```python
from build123d import *

# Parameters (mm, degrees)
F0_R     = 2.25
F0_R_2   = 1.5
F0_R_3   = 3
F0_W     = 71.6
F0_H     = 55.3
F0_W_2   = 30
F0_H_2   = 130
F0_W_3   = 243.84
F0_H_3   = 173
F0_R_4   = 1.75
F1_DEPTH = 3
F2_R     = 10


with BuildPart() as f1:
    # F0 (on Front) → F1 (new body)
    with BuildSketch(Plane.XZ):
        with BuildLine():
            Line((-179.2, 113.305101), (-179.2, 63.305101))
            Line((-179.2, 63.305101), (-163.2, 63.305101))
            Line((-163.2, 63.305101), (-149.2, 63.305101))
            Line((-149.2, 63.305101), (-149.2, 116.305101))
            ThreePointArc((-149.2, 116.305101), (-147.735534, 119.840635), (-144.2, 121.305101))
            Line((-144.2, 121.305101), (-49.2, 121.305101))
            ThreePointArc((-49.2, 121.305101), (-45.664466, 119.840635), (-44.2, 116.305101))
            Line((-44.2, 116.305101), (-44.2, 63.305101))
            Line((-44.2, 63.305101), (-43.607167, 63.305101))
            Line((-43.607167, 63.305101), (-36.2, 63.305101))
            Line((-36.2, 63.305101), (-14.2, 63.305101))
            Line((-14.2, 63.305101), (-14.2, 113.305101))
            ThreePointArc((-14.2, 113.305101), (-18.593398, 123.911702), (-29.2, 128.305101))
            Line((-29.2, 128.305101), (-163.2, 128.305101))
            Line((-163.2, 128.305101), (-164.2, 128.305101))
            ThreePointArc((-164.2, 128.305101), (-174.806602, 123.911702), (-179.2, 113.305101))
        make_face()
        with Locations((-153.7, 70.805101)):
            Circle(F0_R, mode=Mode.SUBTRACT)
        with Locations((-153.704742, 121.805101)):
            Circle(F0_R, mode=Mode.SUBTRACT)
        with Locations((-40.7, 70.805101)):
            Circle(F0_R, mode=Mode.SUBTRACT)
        with Locations((-40.704742, 121.805101)):
            Circle(F0_R, mode=Mode.SUBTRACT)
        with BuildLine():
            Line((-179.2, 63.305101), (-224.2, 63.305101))
            Line((-224.2, 63.305101), (-224.2, -116.694899))
            Line((-224.2, -116.694899), (211.64, -116.694899))
            Line((211.64, -116.694899), (211.64, 63.305101))
            Line((211.64, 63.305101), (-14.2, 63.305101))
            Line((-14.2, 63.305101), (-36.2, 63.305101))
            Line((-36.2, 63.305101), (-36.2, -38.694899))
            Line((-36.2, -38.694899), (-96.871792, -38.694899))
            ThreePointArc((-96.871792, -38.694899), (-94.876352, -39.636759), (-94.064873, -41.68868))
            ThreePointArc((-94.064873, -41.68868), (-99.116794, -43.8772), (-97.257953, -38.694899))
            Line((-97.257953, -38.694899), (-163.2, -38.694899))
            Line((-163.2, -38.694899), (-163.2, 63.305101))
            Line((-163.2, 63.305101), (-179.2, 63.305101))
        make_face()
        with Locations((-204.2, -106.694899)):
            Circle(F0_R_2, mode=Mode.SUBTRACT)
        with Locations((-182.293021, -62.426161)):
            Circle(F0_R_3, mode=Mode.SUBTRACT)
        with Locations((-127.878605, -84.55086)):
            Rectangle(F0_W, F0_H, mode=Mode.SUBTRACT)
        with Locations((-168.293021, -62.443685)):
            Circle(F0_R_3, mode=Mode.SUBTRACT)
        with Locations((-82.145924, -103.675909)):
            Circle(F0_R_3, mode=Mode.SUBTRACT)
        with Locations((-82.184737, -87.675909)):
            Circle(F0_R_3, mode=Mode.SUBTRACT)
        with Locations((-42.651812, -103.716843)):
            Circle(F0_R_3, mode=Mode.SUBTRACT)
        with Locations((-42.690625, -87.716843)):
            Circle(F0_R_3, mode=Mode.SUBTRACT)
        with Locations((-182.38479, -35.251863)):
            Circle(F0_R_3, mode=Mode.SUBTRACT)
        with Locations((-155.771547, -53.774103)):
            Circle(F0_R_3, mode=Mode.SUBTRACT)
        with Locations((-155.810359, -41.774103)):
            Circle(F0_R_3, mode=Mode.SUBTRACT)
        with Locations((-168.38479, -35.269387)):
            Circle(F0_R_3, mode=Mode.SUBTRACT)
        with Locations((-203.2, -24.000519)):
            Rectangle(F0_W_2, F0_H_2, mode=Mode.SUBTRACT)
        with Locations((-97.02606, -53.68868)):
            Circle(F0_R_3, mode=Mode.SUBTRACT)
        with Locations((87.72, -25.194899)):
            Rectangle(F0_W_3, F0_H_3, mode=Mode.SUBTRACT)
        with Locations((-182.422297, 22.783056)):
            Circle(F0_R_3, mode=Mode.SUBTRACT)
        with Locations((-168.422297, 22.765532)):
            Circle(F0_R_3, mode=Mode.SUBTRACT)
        with Locations((-204.2, 53.305101)):
            Circle(F0_R_2, mode=Mode.SUBTRACT)
        with Locations((-203.2, -24.000519)):
            Rectangle(F0_W_2, F0_H_2)
        with Locations((-203.2, -59.000519)):
            Circle(F0_R_4, mode=Mode.SUBTRACT)
        with Locations((-203.2, 5.999481)):
            Circle(F0_R_4, mode=Mode.SUBTRACT)
        with Locations((-127.878605, -84.55086)):
            Rectangle(F0_W, F0_H)
        with Locations((-161.178605, -93.40086)):
            Circle(F0_R_2, mode=Mode.SUBTRACT)
        with Locations((-161.178605, -65.50086)):
            Circle(F0_R_2, mode=Mode.SUBTRACT)
        with Locations((-109.378605, -108.60086)):
            Circle(F0_R_2, mode=Mode.SUBTRACT)
        with Locations((-108.078605, -60.40086)):
            Circle(F0_R_2, mode=Mode.SUBTRACT)
        with BuildLine():
            Line((-149.2, 63.305101), (-163.2, 63.305101))
            Line((-163.2, 63.305101), (-163.2, -38.694899))
            Line((-163.2, -38.694899), (-97.257953, -38.694899))
            ThreePointArc((-97.257953, -38.694899), (-97.064873, -38.68868), (-96.871792, -38.694899))
            Line((-96.871792, -38.694899), (-36.2, -38.694899))
            Line((-36.2, -38.694899), (-36.2, 63.305101))
            Line((-36.2, 63.305101), (-43.607167, 63.305101))
            Line((-43.607167, 63.305101), (-44.2, 63.305101))
            Line((-44.2, 63.305101), (-141.720161, 63.305101))
            Line((-141.720161, 63.305101), (-149.2, 63.305101))
        make_face()
        with Locations((87.72, -25.194899)):
            Rectangle(F0_W_3, F0_H_3)
        with Locations((-20.32, -103.694899)):
            Circle(F0_R_2, mode=Mode.SUBTRACT)
        with Locations((45.72, -103.694899)):
            Circle(F0_R_2, mode=Mode.SUBTRACT)
        with Locations((203.2, -103.694899)):
            Circle(F0_R_2, mode=Mode.SUBTRACT)
        with Locations((0, 51.145101)):
            Circle(F0_R_2, mode=Mode.SUBTRACT)
        with Locations((45.72, 51.145101)):
            Circle(F0_R_2, mode=Mode.SUBTRACT)
        with Locations((203.2, 28.295101)):
            Circle(F0_R_2, mode=Mode.SUBTRACT)
    extrude(amount=F1_DEPTH)

    # F2
    f2_edges = [f1.edges().sort_by_distance(p)[0] for p in [
        (-224.2, -1.5, 63.305101),
        (-224.2, -1.5, -116.694899),
    ]]
    fillet(f2_edges, radius=F2_R)


solid = f1.part
```
CAD build for the part. Positions are in the model's coordinates, mm. Coordinates: 2 decimals unless noted, no trailing zeros. Write each loop counter-clockwise with the first axis right and the second up, starting at its lowest first coordinate (ties: lowest second). Pieces come first, ordered by that corner, then holes.
(1) Cut at A-A, the plane z = 85. List the corners of the cut face in (x, y).
(2) Drill centre lines: probe 1 along Z at (x, y) = (-204.2, -0.85); probe 2 along X at (y, z) = (-1.55, 77); probe 3 along Z at (x, y) = (-104, -0.95). Where is each one in solid material? Low to high.
(3) Flat gauge pins, fed straight in: pin 1 (0.9 mm diameter, centred on x = -193.5, y = -1.5, fed in from +Z); pin 2 (2.5 mm diameter, centred on x = 45.72, z = -103.69, fed in from -Y); pin 3 (1 mm diameter, centred on y = -0.5, z = 95, fed in from +X); pin 4 (0.9 mm diameter, centred on y = -1.5, z = 91.5, fed in from -X). Where does each tip first touch, or does it go through?
(4) Cut at B-B, the plane x = -90. List the corners of the cut face in (y, z), and give its area (3 significant figures).
(5) Cut at C-C, the plane y = -1.6. Count the separate pieces of the cut face and the enclosed holes in it, and give its area (3 significant figures).
Geometry says:
1. outline: (-179.2, -3) - (-149.2, -3) - (-149.2, 0) - (-179.2, 0) - close; (-44.2, -3) - (-14.2, -3) - (-14.2, 0) - (-44.2, 0) - close
2. probe 1: z = -116.69 to -108.19, -105.19 to -60.44, -57.56 to 4.56, 7.44 to 51.81, 54.81 to 63.31
2. probe 2: x = -179.2 to -149.2, -44.2 to -14.2
2. probe 3: z = -116.69 to 63.31, 121.31 to 128.31
3. pin 1: stops at z = 63.31
3. pin 2: passes through
3. pin 3: stops at x = -14.2
3. pin 4: stops at x = -179.2
4. outline: (-3, -116.69) - (0, -116.69) - (0, 63.31) - (-3, 63.31) - close; (-3, 121.31) - (0, 121.31) - (0, 128.31) - (-3, 128.31) - close
4. area: 561 mm2
5. separate pieces: 1
5. enclosed holes: 33
5. area: 82,400 mm2
